Geometry check sheet. Reference: the model listing, model coordinates, mm. A direction names the side the tool comes from. Round coordinates to 2 decimals unless told otherwise and drop trailing zeros. Write each loop counter-clockwise with the first axis right and the second up, starting at its lowest first coordinate (ties: lowest second). Pieces come first, ordered by that corner, then holes. Notation, with made-up numbers: (15, 7.25) -> (68, 7.25) arc R12 cw to (68, 26.25) -> close; hole circle Ø5 at (41, 42). An arc over 180 degrees is marked (long way). Return JSON: item names as keys, results as strings. Group by question number.
from build123d import *

# Parameters (mm, degrees)
SKETCH_1_W                             = 42
SKETCH_1_H                             = 24
SKETCH_1_W_2                           = 23.8
SKETCH_1_H_2                           = 12.8
SG90_WINDOW23P8X12P8_DEPTH             = 3
SG90_MOUNT_SLOTS_REFERENCE_DEPTH       = 25.372115214
SG90_MOUNT_SLOTS_REFERENCE_DEPTH_BACK  = 25.372115214
SKETCH_2_W                             = 2.4
SKETCH_2_H                             = 4
ADAPTER_M3_PAIR12_REFERENCE_DEPTH      = 25.372115214
ADAPTER_M3_PAIR12_REFERENCE_DEPTH_BACK = 25.372115214
SKETCH_3_R                             = 1.7


with BuildPart() as part:
    # 草图1 → SG90_window23p8x12p8 (new body)
    with BuildSketch(Plane.XY):
        Rectangle(SKETCH_1_W, SKETCH_1_H)
        Rectangle(SKETCH_1_W_2, SKETCH_1_H_2, mode=Mode.SUBTRACT)
    extrude(amount=SG90_WINDOW23P8X12P8_DEPTH)

    # 草图2 → SG90_mount_slots_REFERENCE (cut, two sides: drawn at the far end of the back side and taken through both)
    with BuildSketch(Plane.XY.offset(-SG90_MOUNT_SLOTS_REFERENCE_DEPTH_BACK)):
        with Locations((-14, 0)):
            Rectangle(SKETCH_2_W, SKETCH_2_H)
        with Locations((14, 0)):
            Rectangle(SKETCH_2_W, SKETCH_2_H)
    extrude(amount=SG90_MOUNT_SLOTS_REFERENCE_DEPTH + SG90_MOUNT_SLOTS_REFERENCE_DEPTH_BACK, mode=Mode.SUBTRACT)

    # 草图3 → Adapter_M3_pair12_REFERENCE (cut, two sides: drawn at the far end of the back side and taken through both)
    with BuildSketch(Plane.XY.offset(-ADAPTER_M3_PAIR12_REFERENCE_DEPTH_BACK)):
        with Locations((-6, -9)):
            Circle(SKETCH_3_R)
        with Locations((6, -9)):
            Circle(SKETCH_3_R)
    extrude(amount=ADAPTER_M3_PAIR12_REFERENCE_DEPTH + ADAPTER_M3_PAIR12_REFERENCE_DEPTH_BACK, mode=Mode.SUBTRACT)


solid = part.part
1) Tool access check on faces 1 (the face through (0, 8, 3)), 2 (the face through (-15.2, 0, 1)). Record the directions out of +Z, -Z, +X, -X, +Y, -Y that give a thin tool (end or side, any length) a straight path to the whole face; none if there is none.
2) Mould release check, pull along X, two halves, no side actions. Record for faces 3 (the face through (0, 8, 0)), 4 (the face through (-21, 0, 1)), 5 (the face through (0, -6.4, 1)): +X half, -X half, draft (parallel to the pull), parting line (faces both ways), or undercut.
3) Sectioned sample at D-D on z = 2.4. Enter the section's corners in (x, y), and give its area (3 significant figures).
4) Sectioned sample at A-A on x = 10. Enter the section's corners in (y, z), and give its area (3 significant figures).
5) Sectioned sample at C-C on x = -6. Enter the section's corners in (y, z), and give its area (3 significant figures).
6) Material ranges on probe 1 along Y at (x, z) = (-6, 1.65); probe 2 along X at (y, z) = (-9, 1.85); probe 3 along X at (y, z) = (-1.5, 2.25), recorded low to high. Write a range as [from, to].
7) Sectioned sample at B-B on y = -9. Enter the section's corners in (x, z).
8) Go/stop test with a flat-tipped pin: P1, Ø4, axis at x = -4, y = -3.5, coming from the -Z side. Record where the tip stops, or that it passes through.
Evaluation:
{
 "1": {"face 1": "+Z, +X, -X, +Y, -Y", "face 2": "+Z, -Z"},
 "2": {"face 3": "draft", "face 4": "-X half", "face 5": "undercut"},
 "3": {"outline": "(-21, -12) -> (21, -12) -> (21, 12) -> (-21, 12) -> close; hole (-15.2, -2) -> (-12.8, -2) -> (-12.8, 2) -> (-15.2, 2) -> close; hole (-11.9, -6.4) -> (11.9, -6.4) -> (11.9, 6.4) -> (-11.9, 6.4) -> close; hole circle Ø3.4 at (-6, -9); hole circle Ø3.4 at (6, -9); hole (12.8, -2) -> (15.2, -2) -> (15.2, 2) -> (12.8, 2) -> close", "area": "666 mm2"},
 "4": {"outline": "(-12, 0) -> (-6.4, 0) -> (-6.4, 3) -> (-12, 3) -> close; (6.4, 0) -> (12, 0) -> (12, 3) -> (6.4, 3) -> close", "area": "33.6 mm2"},
 "5": {"outline": "(-12, 0) -> (-10.7, 0) -> (-10.7, 3) -> (-12, 3) -> close; (-7.3, 0) -> (-6.4, 0) -> (-6.4, 3) -> (-7.3, 3) -> close; (6.4, 0) -> (12, 0) -> (12, 3) -> (6.4, 3) -> close", "area": "23.4 mm2"},
 "6": {"probe 1": "y = [-12, -10.7], [-7.3, -6.4], [6.4, 12]", "probe 2": "x = [-21, -7.7], [-4.3, 4.3], [7.7, 21]", "probe 3": "x = [-21, -15.2], [-12.8, -11.9], [11.9, 12.8], [15.2, 21]"},
 "7": {"outline": "(-21, 0) -> (-7.7, 0) -> (-7.7, 3) -> (-21, 3) -> close; (-4.3, 0) -> (4.3, 0) -> (4.3, 3) -> (-4.3, 3) -> close; (7.7, 0) -> (21, 0) -> (21, 3) -> (7.7, 3) -> close"},
 "8": {"P1": "passes through"}
}
